Source: three-view drawing plus pictorial views. Frame: mm from the lowest corner of the part. A direction names the side the tool comes from. Coordinates: 2 decimals unless noted, no trailing zeros. Write each loop counter-clockwise with the first axis right and the second up, starting at its lowest first coordinate (ties: lowest second). Pieces come first, ordered by that corner, then holes. Notation, with made-up numbers: (-0.5, -31.75) - (17.5, -31.75) arc R28 cw to (17.5, 0.25) - close; hole circle Ø8 at (-20.5, 5). An arc over 180 degrees is marked (long way). Put each result on its own line as item: value.
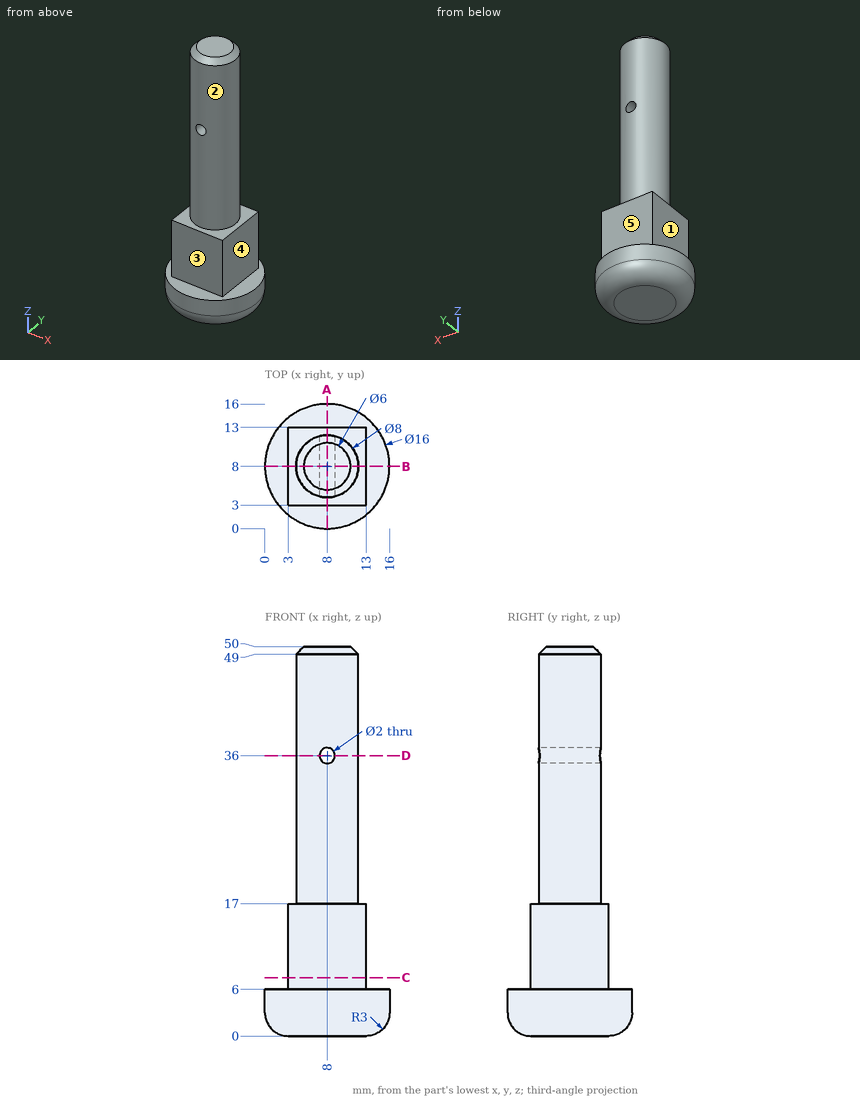
1. Ray query, probe 1 along Z at (x, y) = (8, 9.5); probe 2 along Z at (x, y) = (4.75, 5); probe 3 along X at (y, z) = (6.5, 36). Return the intervals inside material, ascending. Write a range as from..to.
Answer below:
probe 1: z = 0..35, 37..50
probe 2: z = 0..17
probe 3: x = 4.29..7, 9..11.71
2. Section query A-A (x = 8). Return loops of the section in (y, z).
Answer below:
outline: (0, 3) arc R3 ccw to (3, 0) - (13, 0) arc R3 ccw to (16, 3) - (16, 6) - (13, 6) - (13, 17) - (12, 17) - (12, 35) - (4, 35) - (4, 17) - (3, 17) - (3, 6) - (0, 6) - close; (4, 37) - (12, 37) - (12, 49) - (11, 50) - (5, 50) - (4, 49) - close
3. Section query C-C (z = 7.5). Return loops of the section in (x, y).
Answer below:
outline: (3, 3) - (13, 3) - (13, 13) - (3, 13) - close
4. Section query D-D (z = 36). Return loops of the section in (x, y), then the cut area to 3 significant figures.
Answer below:
outline: (7, 4.13) - (7, 11.87) arc R4 ccw to start; (9, 4.13) arc R4 ccw to (9, 11.87) - close
area: 34.4 mm²
5. Set-up query: the marked faces 1, 2, 3, 4 and 5. Return all of +Z, -Z, +X, -X, +Y, -Y with unobstructed straight access to the full face (end or side cutting, diameter ignored); none if empty.
Answer below:
face 1: +Z, -X, +Y, -Y
face 2: +Z
face 3: +Z, +X, -X, -Y
face 4: +Z, +X, +Y, -Y
face 5: +Z, +X, -X, +Y
6. Section query B-B (y = 8). Return loops of the section in (x, z), then the cut area to 3 significant figures.
Answer below:
outline: (0, 3) arc R3 ccw to (3, 0) - (13, 0) arc R3 ccw to (16, 3) - (16, 6) - (13, 6) - (13, 17) - (12, 17) - (12, 49) - (11, 50) - (5, 50) - (4, 49) - (4, 17) - (3, 17) - (3, 6) - (0, 6) - close; hole circle Ø2 at (8, 36)
area: 462 mm²
7. Pin query (flat end, axial travel): pin 1 Ø8 at (y, z) = (2, 23) entering from +X; pin 2 Ø2 at (x, y) = (4.5, 5.5) entering from +Z; pin 3 Ø5 at (y, z) = (3.5, 35) entering from -X. Return the tip coordinate at first contact, or that it passes through.
Answer below:
pin 1: stops at x = 11.46
pin 2: stops at z = 49.7
pin 3: stops at x = 4.54
